For this review, take the finished solid that the model builds, in its own axes (mm). A direction names the side the tool comes from. Give positions to 0.01 mm unless a question says otherwise; leave off trailing zeros. Order: outer loops, then holes, each group sorted by start corner. A loop starts at its lowest first (then second) coordinate and runs counter-clockwise, first axis right, second up.
from build123d import *

# Parameters (mm, degrees)
SKETCH1_R           = 76
BOSS_EXTRUDE1_DEPTH = 75


with BuildPart() as part:
    # Sketch1 → Boss-Extrude1 (new body)
    with BuildSketch(Plane.XY):
        Circle(SKETCH1_R)
        with BuildLine():
            Line((-9, 31.228992939), (-9, 36.8))
            Line((-9, 36.8), (9, 36.8))
            Line((9, 36.8), (9, 31.228992939))
            ThreePointArc((9, 31.228992939), (0, -32.5), (-9, 31.228992939))
        make_face(mode=Mode.SUBTRACT)
    extrude(amount=BOSS_EXTRUDE1_DEPTH)


solid = part.part
1) We need section A-A on y = 0. Give the boundary of the cut face in (x, z), then the cut area to 4 significant figures.
Answer sheet:
outline: (-76, 0) - (-32.5, 0) - (-32.5, 75) - (-76, 75) - close; (32.5, 0) - (76, 0) - (76, 75) - (32.5, 75) - close
area: 6,525 mm2
2) Draft analysis for pull direction Y (two halves, no side actions). For faces 3 (the face through (0, 36.8, 37)), 4 (the face through (35.069, -67.425, 36.975)), 5 (the face through (-1, -33, 75)), 6 (the face through (-9, 34, 37)), state which applies: +Y half, -Y half, draft (parallel to the pull), parting line (faces both ways), or undercut.
Answer sheet:
face 3: undercut
face 4: parting line
face 5: draft
face 6: undercut
3) We need section C-C on z = 16. Give the boundary of the cut face in (x, y), then the cut area to 3 significant figures.
Answer sheet:
outline: circle Ø152 at (0, 0); hole (-9, 31.23) arc R32.5 ccw (long way) to (9, 31.23) - (9, 36.8) - (-9, 36.8) - close
area: 14,700 mm2
4) Tool access review of faces 1 (the face through (9, 34, 37)), 2 (the face through (-1, -33, 0)): name each direction out of +Z, -Z, +X, -X, +Y, -Y from which nothing blocks a thin tool from reaching the whole face with its end or side.
Answer sheet:
face 1: +Z, -Z
face 2: -Z, +X, -X, +Y, -Y
5) We need section B-B on x = 0. Give the boundary of the cut face in (y, z), then the cut area to 3 significant figures.
Answer sheet:
outline: (-76, 0) - (-32.5, 0) - (-32.5, 75) - (-76, 75) - close; (36.8, 0) - (76, 0) - (76, 75) - (36.8, 75) - close
area: 6,200 mm2
6) To check wall thickness, follow line 1 (Y direction, x = 0, z = 19.5); line 2 (Y direction, x = -10, z = 6); line 3 (X direction, y = -15.5, z = 29). State the ranges of each line that lie inside material, in increasing order.
Answer sheet:
line 1: y = -76 to -32.5, 36.8 to 76
line 2: y = -75.34 to -30.92, 30.92 to 75.34
line 3: x = -74.4 to -28.57, 28.57 to 74.4
7) We need section D-D on y = -45. Give the boundary of the cut face in (x, z).
Answer sheet:
outline: (-61.25, 0) - (61.25, 0) - (61.25, 75) - (-61.25, 75) - close
8) Clearance check with flat-ended pins moving along their axes: pin 1 (3 mm diameter, centred on y = 24, z = 42, fed in from +X); pin 2 (5.5 mm diameter, centred on x = 0.5, z = 35.5, fed in from -Y); pin 3 (3 mm diameter, centred on y = 35, z = 52, fed in from +X). State where each tip first meets the part, or that it passes through.
Answer sheet:
pin 1: stops at x = 72.59
pin 2: stops at y = -76
pin 3: stops at x = 68.22
